from build123d import *

# Parameters (mm, degrees)
F0_W          = 40
F0_H          = 70
F1_DEPTH      = 7
F2_R          = 0.7899610996
F2_R_2        = 0.7879667618
F2_R_3        = 1.8073925599
F2_R_4        = 0.8167266128
F3_DEPTH      = 10
F5_DEPTH      = 12
F7_DEPTH      = 13
F8_R          = 3.7758905803
F9_DEPTH      = 1
F10_W         = 14.9725805968
F10_H         = 2.3034736514
F10_R         = 1.22160092
F11_DEPTH     = 2
F12_T1_DEPTH  = 32
F13_R         = 5
F14_R         = 5
F15_T1_DEPTH  = 32
F16_T1_DEPTH  = 60
F16_T3_DEPTH  = 30
F16_T6_ANGLE  = 90
F16_T8_ANGLE  = 89.9999999974
F16_T10_ANGLE = 89.9999999974
F16_T12_ANGLE = 90
F17_T1_DEPTH  = 60
F17_T3_DEPTH  = 30
F17_T6_ANGLE  = 90
F17_T8_ANGLE  = 89.9999999974
F17_T10_ANGLE = 89.9999999974
F17_T12_ANGLE = 90


# Not quite as in the source:
# - a fillet or chamfer that OpenCascade refuses, or shapes differently, is made with other operations: its cross-section is extruded or revolved along the edge and cut away or added
# - ends of sketch curves that miss each other by under 0.0002 mm in the source are joined


with BuildPart() as f1:
    # F0 (on Top) → F1 (new body)
    with BuildSketch(Plane.XY):
        with Locations((20, 35)):
            Rectangle(F0_W, F0_H)
    extrude(amount=F1_DEPTH)

    # F2 (on face) → F3 (cut)
    with BuildSketch(Plane.XZ):
        with Locations((15.5336856842, 3.5)):
            Circle(F2_R)
        with BuildLine():
            Line((20.5575972795, 4.779751625), (18.0456396192, 4.779751625))
            ThreePointArc((18.0456396192, 4.779751625), (16.7658879943, 3.5), (18.0456396192, 2.220248375))
            Line((18.0456396192, 2.220248375), (20.5575972795, 2.220248375))
            ThreePointArc((20.5575972795, 2.220248375), (21.8373489045, 3.5), (20.5575972795, 4.779751625))
        make_face()
        with Locations((27.6224724948, 3.5)):
            Circle(F2_R_2)
        with Locations((23.0695530772, 3.5)):
            Circle(F2_R)
        with Locations((29.6224724948, 3.5)):
            Circle(F2_R_2)
        with Locations((31.6224724948, 3.5)):
            Circle(F2_R_2)
        with Locations((33.6224724948, 3.5)):
            Circle(F2_R_2)
        with Locations((35.6224724948, 3.5)):
            Circle(F2_R_2)
        with Locations((37.6224724948, 3.5)):
            Circle(F2_R_2)
        with Locations((5.3267837502, 3.5)):
            Circle(F2_R_3)
        with Locations((8.1548150629, 3.5)):
            Circle(F2_R_4)
    extrude(amount=-F3_DEPTH, mode=Mode.SUBTRACT)

    # F4 (on face) → F5 (cut)
    with BuildSketch(Plane.YZ.offset(40)):
        with BuildLine():
            Line((45.7730665803, 4.75), (41.0204045475, 4.75))
            ThreePointArc((41.0204045475, 4.75), (39.7704045475, 3.5000009306), (41.0204026863, 2.25))
            Line((41.0204026863, 2.25), (45.7730665803, 2.25))
            ThreePointArc((45.7730665803, 2.25), (47.0230665803, 3.5), (45.7730665803, 4.75))
        make_face()
    extrude(amount=-F5_DEPTH, mode=Mode.SUBTRACT)

    # F6 (on face) → F7 (join)
    with BuildSketch(Plane.YZ.offset(28)):
        with BuildLine():
            Line((45.7748817965, 4.3017610189), (41.022244125, 4.312521164))
            ThreePointArc((41.022244125, 4.312521164), (41.0213243392, 4.3125248082), (41.0204045475, 4.3125253288))
            ThreePointArc((41.0204045475, 4.3125253288), (40.2078792186, 3.5000009306), (41.0204026863, 2.6874746712))
            ThreePointArc((41.0204026863, 2.6874746712), (41.0213234086, 2.6874751907), (41.0222441297, 2.6874767536))
            Line((41.0222441297, 2.6874767536), (45.7748817965, 2.6982389853))
            ThreePointArc((45.7748817965, 2.6982389853), (46.5748296498, 3.5), (45.7748817965, 4.3017610189))
        make_face()
    extrude(amount=F7_DEPTH)

    # F8 (on face) → F9 (cut)
    with BuildSketch(Plane.XY.offset(7)):
        with Locations((20, 8.0621577799)):
            Circle(F8_R)
    extrude(amount=-F9_DEPTH, mode=Mode.SUBTRACT)

    # F10 (on face) → F11 (cut)
    with BuildSketch(Plane.XY.offset(7)):
        with Locations((19.9095932767, 66.3465745747)):
            Rectangle(F10_W, F10_H)
        with Locations((9.5746694133, 66.4882957935)):
            Circle(F10_R)
    extrude(amount=-F11_DEPTH, mode=Mode.SUBTRACT)

    # F12: fillet of radius 5 on 1 edges, made by hand

    # F12_s2 → F12_t1 (cut)
    with BuildSketch(Plane.XY.offset(-12.5)):
        with BuildLine():
            ThreePointArc((0, 5), (1.4644660941, 1.4644660941), (5, 0))
            Line((5, 0), (0, 0))
            Line((0, 0), (0, 5))
        make_face()
    extrude(amount=F12_T1_DEPTH, mode=Mode.SUBTRACT)

    # F13
    f13_edges = [f1.edges().sort_by_distance(p)[0] for p in [
        (0, 70, 3.5),
    ]]
    fillet(f13_edges, radius=F13_R)

    # F14
    f14_edges = [f1.edges().sort_by_distance(p)[0] for p in [
        (40, 70, 3.5),
    ]]
    fillet(f14_edges, radius=F14_R)

    # F15: fillet of radius 5 on 1 edges, made by hand

    # F15_s2 → F15_t1 (cut)
    with BuildSketch(Plane.XY.offset(-12.5)):
        with BuildLine():
            ThreePointArc((40, 5), (38.5355339059, 1.4644660941), (35, 0))
            Line((35, 0), (40, 0))
            Line((40, 0), (40, 5))
        make_face()
    extrude(amount=F15_T1_DEPTH, mode=Mode.SUBTRACT)

    # F16: fillet of radius 2 on 2 edges, made by hand

    # F16_s2 → F16_t1 (cut)
    with BuildSketch(Plane.XZ.offset(-65)):
        with BuildLine():
            ThreePointArc((40, 5), (39.4142135624, 6.4142135624), (38, 7))
            Line((38, 7), (40, 7))
            Line((40, 7), (40, 5))
        make_face()
        with BuildLine():
            ThreePointArc((0, 5), (0.5857864376, 6.4142135624), (2, 7))
            Line((2, 7), (0, 7))
            Line((0, 7), (0, 5))
        make_face()
    extrude(amount=F16_T1_DEPTH, mode=Mode.SUBTRACT)

    # F16_s4 → F16_t3 (cut)
    with BuildSketch(Plane.YZ.offset(5)):
        with BuildLine():
            ThreePointArc((0, 5), (0.5857864376, 6.4142135624), (2, 7))
            Line((2, 7), (0, 7))
            Line((0, 7), (0, 5))
        make_face()
        with BuildLine():
            ThreePointArc((70, 5), (69.4142135624, 6.4142135624), (68, 7))
            Line((68, 7), (70, 7))
            Line((70, 7), (70, 5))
        make_face()
    extrude(amount=F16_T3_DEPTH, mode=Mode.SUBTRACT)

    # F16_s5 → F16_t6 (revolve, cut)
    with BuildSketch(Plane.XZ.offset(-65)):
        with BuildLine():
            ThreePointArc((0, 5), (0.5857864376, 6.4142135624), (2, 7))
            Line((2, 7), (0, 7))
            Line((0, 7), (0, 5))
        make_face()
    revolve(axis=Axis((5, 65, 7), (0, 0, -1)), revolution_arc=F16_T6_ANGLE, mode=Mode.SUBTRACT)

    # F16_s7 → F16_t8 (revolve, cut)
    with BuildSketch(Plane.YZ.offset(5.0000000001)):
        with BuildLine():
            ThreePointArc((0, 5), (0.5857864376, 6.4142135624), (2, 7))
            Line((2, 7), (0, 7))
            Line((0, 7), (0, 5))
        make_face()
    revolve(axis=Axis((5.0000000001, 5.0000000001, 7), (0, 0, -1)), revolution_arc=F16_T8_ANGLE, mode=Mode.SUBTRACT)

    # F16_s9 → F16_t10 (revolve, cut)
    with BuildSketch(Plane.XZ.offset(-5.0000000001)):
        with BuildLine():
            ThreePointArc((40, 5), (39.4142135624, 6.4142135624), (38, 7))
            Line((38, 7), (40, 7))
            Line((40, 7), (40, 5))
        make_face()
    revolve(axis=Axis((34.9999999999, 5.0000000001, 7), (0, 0, -1)), revolution_arc=F16_T10_ANGLE, mode=Mode.SUBTRACT)

    # F16_s11 → F16_t12 (revolve, cut)
    with BuildSketch(Plane.YZ.offset(35)):
        with BuildLine():
            ThreePointArc((70, 5), (69.4142135624, 6.4142135624), (68, 7))
            Line((68, 7), (70, 7))
            Line((70, 7), (70, 5))
        make_face()
    revolve(axis=Axis((35, 65, 7), (0, 0, -1)), revolution_arc=F16_T12_ANGLE, mode=Mode.SUBTRACT)

    # F17: fillet of radius 2 on 8 edges, made by hand

    # F17_s2 → F17_t1 (cut)
    with BuildSketch(Plane.XZ.offset(-65)):
        with BuildLine():
            ThreePointArc((2, 0), (0.5857864376, 0.5857864376), (0, 2))
            Line((0, 2), (0, 0))
            Line((0, 0), (2, 0))
        make_face()
        with BuildLine():
            ThreePointArc((38, 0), (39.4142135624, 0.5857864376), (40, 2))
            Line((40, 2), (40, 0))
            Line((40, 0), (38, 0))
        make_face()
    extrude(amount=F17_T1_DEPTH, mode=Mode.SUBTRACT)

    # F17_s4 → F17_t3 (cut)
    with BuildSketch(Plane.YZ.offset(5)):
        with BuildLine():
            ThreePointArc((2, 0), (0.5857864376, 0.5857864376), (0, 2))
            Line((0, 2), (0, 0))
            Line((0, 0), (2, 0))
        make_face()
        with BuildLine():
            ThreePointArc((68, 0), (69.4142135624, 0.5857864376), (70, 2))
            Line((70, 2), (70, 0))
            Line((70, 0), (68, 0))
        make_face()
    extrude(amount=F17_T3_DEPTH, mode=Mode.SUBTRACT)

    # F17_s5 → F17_t6 (revolve, cut)
    with BuildSketch(Plane.YZ.offset(35)):
        with BuildLine():
            ThreePointArc((68, 0), (69.4142135624, 0.5857864376), (70, 2))
            Line((70, 2), (70, 0))
            Line((70, 0), (68, 0))
        make_face()
    revolve(axis=Axis((35, 65, 0), (0, 0, -1)), revolution_arc=F17_T6_ANGLE, mode=Mode.SUBTRACT)

    # F17_s7 → F17_t8 (revolve, cut)
    with BuildSketch(Plane.XZ.offset(-5.0000000001)):
        with BuildLine():
            ThreePointArc((38, 0), (39.4142135624, 0.5857864376), (40, 2))
            Line((40, 2), (40, 0))
            Line((40, 0), (38, 0))
        make_face()
    revolve(axis=Axis((34.9999999999, 5.0000000001, 0), (0, 0, -1)), revolution_arc=F17_T8_ANGLE, mode=Mode.SUBTRACT)

    # F17_s9 → F17_t10 (revolve, cut)
    with BuildSketch(Plane.YZ.offset(5.0000000001)):
        with BuildLine():
            ThreePointArc((2, 0), (0.5857864376, 0.5857864376), (0, 2))
            Line((0, 2), (0, 0))
            Line((0, 0), (2, 0))
        make_face()
    revolve(axis=Axis((5.0000000001, 5.0000000001, 0), (0, 0, -1)), revolution_arc=F17_T10_ANGLE, mode=Mode.SUBTRACT)

    # F17_s11 → F17_t12 (revolve, cut)
    with BuildSketch(Plane.XZ.offset(-65)):
        with BuildLine():
            ThreePointArc((2, 0), (0.5857864376, 0.5857864376), (0, 2))
            Line((0, 2), (0, 0))
            Line((0, 0), (2, 0))
        make_face()
    revolve(axis=Axis((5, 65, 0), (0, 0, -1)), revolution_arc=F17_T12_ANGLE, mode=Mode.SUBTRACT)


solid = f1.part
Part model, mm, in its own coordinate system. A direction names the side the tool comes from. Give positions to 0.01 mm unless a question says otherwise; leave off trailing zeros. Loops run counter-clockwise (first coordinate to the right, second up) from the corner with the lowest first, then second, coordinate; pieces in that order, holes last.
(1) 3-axis set-ups, long thin cutter, end or side, ignore diameter. For faces 1 (the cylindrical face through (34.409, 46.575, 3.482)), 2 (the cylindrical face through (28.35, 4.93, 3.2)), 3 (the flat face through (20, 67.498, 6)): which of +Z, -Z, +X, -X, +Y, -Y reach the whole face in a straight line?
Return value:
face 1: +X
face 2: -Y
face 3: +Z
(2) Pin check, flat tips, straight feed: pin 1 (1.3 mm diameter, centred on x = 18, z = 3.5, fed in from -Y); pin 2 (2 mm diameter, centred on y = 66, z = 6, fed in from +X); pin 3 (1.3 mm diameter, centred on x = 37.5, z = 3, fed in from -Y). Stop position of each tip, or through.
Return value:
pin 1: stops at y = 10
pin 2: stops at x = 39.97
pin 3: stops at y = 0.35
(3) Band-saw the part on B-B (y = 53.5). Write the cut outline in (x, z), and give its area (3 significant figures).
Return value:
outline: (0, 2) arc R2 ccw to (2, 0) - (38, 0) arc R2 ccw to (40, 2) - (40, 5) arc R2 ccw to (38, 7) - (2, 7) arc R2 ccw to (0, 5) - close
area: 277 mm2
(4) Drill centre lines: line 1 along Y through (x, z) = (17, 5.25); line 2 along Y through (x, z) = (21, 2.75); line 3 along X through (y, z) = (44, 5.25). Where is each one in solid material? Low to high.
Return value:
line 1: y = 0.02 to 65.19, 67.5 to 69.98
line 2: y = 10 to 70
line 3: x = 0.02 to 39.98
(5) Pull direction Z, two halves, no side cores. Call faces 4 (the flat face through (20, 70, 3)), 5 (the cylindrical face through (36.835, 5.107, 3.535)), 6 (the cylindrical face through (19.79, 0.57, 6.4)): pulls with the +Z half, pulls with the -Z half, needs draft (parallel to the pull), parting line crosses it, or undercut.
Return value:
face 4: needs draft
face 5: undercut
face 6: pulls with the +Z half
(6) Band-saw the part on A-A (y = 9). Count the separate pieces of the cut face and the enclosed holes in it, and give its area (3 significant figures).
Return value:
separate pieces: 1
enclosed holes: 11
area: 230 mm2
